CAD build for the part. Positions are in the model's coordinates, mm. Face numbers are marked on the shaded views. Give positions to 0.01 mm unless a question says otherwise; leave off trailing zeros. Write each loop counter-clockwise with the first axis right and the second up, starting at its lowest first coordinate (ties: lowest second). Pieces come first, ordered by that corner, then holes. Notation, with made-up numbers: (21, -6.75) - (58, -6.75) arc R30 ccw to (58, 27.25) - close; hole circle Ø6 at (62, 89.25). An arc over 180 degrees is marked (long way). Put each result on its own line as item: value. Start each with the question number.
1. Cut at D-D on y = 4.5. List the corners of the cut face in (x, z), and give its area (3 significant figures).
2. Drop flat-ended pins along their axis: pin 1 (10 mm diameter, centred on x = -10.5, z = -14.5, fed in from +Y); pin 2 (1.5 mm diameter, centred on y = 1, z = -4, fed in from -X); pin 3 (1.5 mm diameter, centred on y = 3.5, z = -14.5, fed in from +X); pin 4 (1.9 mm diameter, centred on x = 2.5, y = 1.5, fed in from -Z). Give the stop position or say it passes through.
3. Wall check: line 1 (Y direction, x = 5.5, z = -7.25); line 2 (Z direction, x = 3, y = 2); line 3 (Z direction, x = -2, y = 1.25). Give the ranges that are in metal, low to high.
4. Cut at A-A on y = 2. List the corners of the cut face in (x, z).
5. Cut at C-C on x = -3. List the corners of the cut face in (y, z), and give its area (3 significant figures).
6. Cut at B-B on z = -7.25. List the corners of the cut face in (x, y).
7. Mould opens along X. For the marked faces 1, 2, 3 and 4 say: +X half, -X half, draft (parallel to the pull), parting line (faces both ways), or undercut.
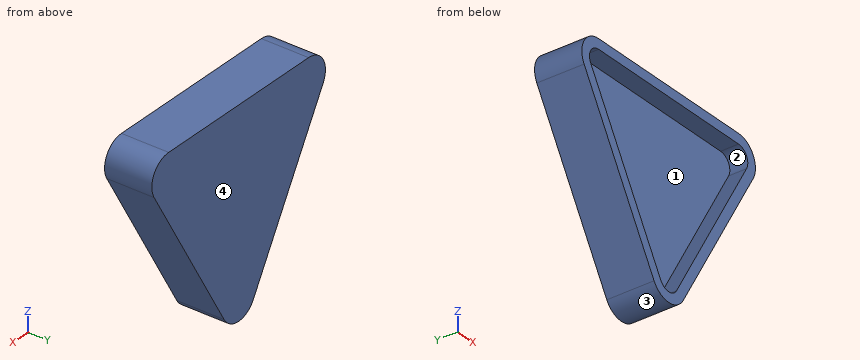
from build123d import *

# Parameters (mm, degrees)
BOSS_EXTRUDE1_DEPTH = 6.35
CUT_EXTRUDE1_DEPTH  = 2.413


with BuildPart() as part:
    # Sketch1 → Boss-Extrude1 (new body)
    with BuildSketch(Plane(origin=(0, 0, 0), x_dir=(1, 0, 0), z_dir=(0, 1, 0))):
        with BuildLine():
            Line((2.54, 25.521030316), (14.734573723, 4.399409051))
            ThreePointArc((14.734573723, 4.399409051), (14.734573723, 1.466469684), (12.194573723, 0))
            Line((12.194573723, 0), (-12.194573723, 0))
            ThreePointArc((-12.194573723, 0), (-14.734573723, 1.466469684), (-14.734573723, 4.399409051))
            Line((-14.734573723, 4.399409051), (-2.54, 25.521030316))
            ThreePointArc((-2.54, 25.521030316), (0, 26.9875), (2.54, 25.521030316))
        make_face()
    extrude(amount=BOSS_EXTRUDE1_DEPTH)

    # Sketch2 → Cut-Extrude1 (cut)
    with BuildSketch(Plane.XZ):
        with BuildLine():
            Line((-13.579728847, -3.732659051), (-1.385155124, -24.854280316))
            ThreePointArc((-1.385155124, -24.854280316), (0, -25.654), (1.385155124, -24.854280316))
            Line((1.385155124, -24.854280316), (13.579728847, -3.732659051))
            ThreePointArc((13.579728847, -3.732659051), (13.579728847, -2.133219684), (12.194573723, -1.3335))
            Line((12.194573723, -1.3335), (-12.194573723, -1.3335))
            ThreePointArc((-12.194573723, -1.3335), (-13.579728847, -2.133219684), (-13.579728847, -3.732659051))
        make_face()
    extrude(amount=-CUT_EXTRUDE1_DEPTH, mode=Mode.SUBTRACT)


solid = part.part
Report:
1. outline: (-14.73, -4.4) - (-2.54, -25.52) arc R2.93 ccw to (2.54, -25.52) - (14.73, -4.4) arc R2.93 ccw to (12.19, 0) - (-12.19, 0) arc R2.93 ccw to start
1. area: 499 mm²
2. pin 1: stops at y = 6.35
2. pin 2: stops at x = -15.11
2. pin 3: stops at x = 9.34
2. pin 4: stops at z = -26.54
3. line 1: y = 2.41 to 6.35
3. line 2: z = -24.72 to -22.06, -1.33 to 0
3. line 3: z = -26.2 to -23.79, -1.33 to 0
4. outline: (-14.73, -4.4) - (-2.54, -25.52) arc R2.93 ccw to (2.54, -25.52) - (14.73, -4.4) arc R2.93 ccw to (12.19, 0) - (-12.19, 0) arc R2.93 ccw to start; hole (-13.58, -3.73) - (-1.39, -24.85) arc R1.6 ccw to (1.39, -24.85) - (13.58, -3.73) arc R1.6 ccw to (12.19, -1.33) - (-12.19, -1.33) arc R1.6 ccw to start
5. outline: (0, -24.72) - (6.35, -24.72) - (6.35, 0) - (0, 0) - (0, -1.33) - (2.41, -1.33) - (2.41, -22.06) - (0, -22.06) - close
5. area: 107 mm²
6. outline: (-13.09, 0) - (-11.55, 0) - (-11.55, 2.41) - (11.55, 2.41) - (11.55, 0) - (13.09, 0) - (13.09, 6.35) - (-13.09, 6.35) - close
7. face 1: undercut
7. face 2: undercut
7. face 3: parting line
7. face 4: draft
